Input: part model. Units: mm. Frame: model coordinates. Face numbers are marked on the shaded views. A direction names the side the tool comes from. Give positions to 0.01 mm unless a question says otherwise; leave off trailing zeros. Loops run counter-clockwise (first coordinate to the right, second up) from the corner with the lowest first, then second, coordinate; pieces in that order, holes last. Notation, with made-up numbers: (-10.75, -21.5) -> (30.25, -21.5) arc R18 ccw to (30.25, 5.5) -> close; hole circle Ø10 at (-32.5, -28). An arc over 180 degrees is marked (long way). Use CSV: the item, a comma, the result in double quotes.
```python
from build123d import *

# Parameters (mm, degrees)
BOSS_EXTRUDE1_DEPTH  = 2.54
SKETCH2_R            = 1.27
CUT_EXTRUDE1_DEPTH   = 5.334
SKETCH3_W            = 13.462
SKETCH3_H            = 27.94
BOSS_EXTRUDE2_DEPTH  = 2.54
BOSS_EXTRUDE3_DEPTH  = 13.462
BOSS_EXTRUDE7_DEPTH  = 1.27
BOSS_EXTRUDE12_DEPTH = 1.27


with BuildPart() as part:
    # Sketch1 → Boss-Extrude1 (new body)
    with BuildSketch(Plane(origin=(0, 0, 0), x_dir=(1, 0, 0), z_dir=(0, 1, 0))):
        Polygon((0, 0), (6.731, 0), (6.731, 38.1), (-6.731, 38.1), (-6.731, 0), align=None)
    extrude(amount=BOSS_EXTRUDE1_DEPTH)

    # Sketch2 → Cut-Extrude1 (cut)
    with BuildSketch(Plane(origin=(0, 2.54, 0), x_dir=(1, 0, 0), z_dir=(0, 1, 0))):
        with Locations(Location((0, 25.429147729, 0), (0, 0, 270))):
            Circle(SKETCH2_R)
        with Locations(Location((0, 12.776292729, 0), (0, 0, 270))):
            Circle(SKETCH2_R)
    extrude(amount=-CUT_EXTRUDE1_DEPTH, mode=Mode.SUBTRACT)

    # Sketch3 → Boss-Extrude2 (add)
    with BuildSketch(Plane.XY):
        with Locations((0, -11.43)):
            Rectangle(SKETCH3_W, SKETCH3_H)
    extrude(amount=-BOSS_EXTRUDE2_DEPTH)

    # Sketch4 → Boss-Extrude3 (add)
    with BuildSketch(Plane.ZY.offset(6.731)):
        with BuildLine():
            Line((0, -25.4), (-2.54, -25.4))
            ThreePointArc((-2.54, -25.4), (9.398, -37.338), (21.336, -25.4))
            Line((21.336, -25.4), (18.796, -25.4))
            ThreePointArc((18.796, -25.4), (9.398, -34.798), (0, -25.4))
        make_face()
    extrude(amount=-BOSS_EXTRUDE3_DEPTH)

    # Sketch8 → Boss-Extrude7 (add)
    with BuildSketch(Plane(origin=(6.731, 0, 0), x_dir=(0, 0, -1), z_dir=(1, 0, 0))):
        Polygon((2.54, -22.86), (20.32, 0), (12.400973841, 0), (2.54, -12.678394938), align=None)
    extrude(amount=-BOSS_EXTRUDE7_DEPTH)

    # Sketch9 → Boss-Extrude12 (add)
    with BuildSketch(Plane.ZY.offset(6.731)):
        Polygon((-2.54, -12.678394938), (-2.54, -22.86), (-20.32, 0), (-12.400973841, 0), align=None)
    extrude(amount=-BOSS_EXTRUDE12_DEPTH)


solid = part.part
```
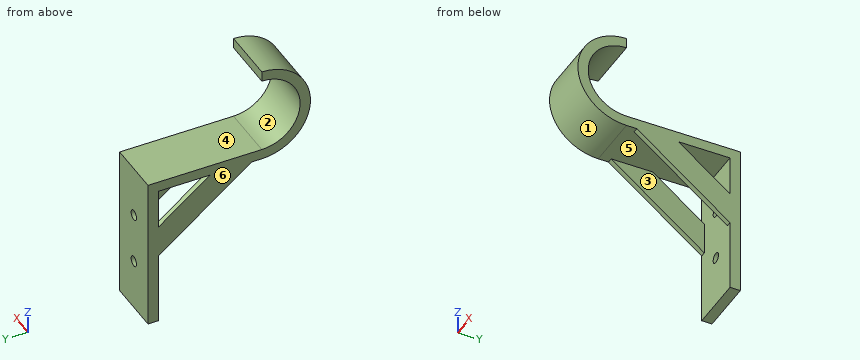
1) Reachability of the marked faces 5 and 6 from +Z, -Z, +X, -X, +Y, -Y: full face, straight path, thin tool, end or side. Return the list, or none.
From the geometry:
face 5,"none"
face 6,"+Z, -Z, -X, +Y, -Y"
2) Contact query for flat-ended pins moving along their axis: pin 1 (8 mm diameter, centred on x = -4, y = -16, fed in from -Z); pin 2 (1.5 mm diameter, centred on x = 0.5, z = 9, fed in from +Y); pin 3 (8 mm diameter, centred on x = 5, y = -9, fed in from -Z). Output: stop coordinate, or through.
From the geometry:
pin 1,"stops at z = -10.77"
pin 2,"stops at y = -34.73"
pin 3,"stops at z = -16.41"
3) Mould query, pull axis Z, two halves, no side actions, for the marked faces 1, 2, 3 and 4. Classes: pulls with the +Z half, pulls with the -Z half, needs draft (parallel to the pull), parting line crosses it, or undercut.
From the geometry:
face 1,"parting line crosses it"
face 2,"undercut"
face 3,"needs draft"
face 4,"pulls with the +Z half"
4) Section query D-D (y = -16.5). Return loops of the section in (x, z).
From the geometry:
outline,"(-6.73, -7.49) -> (-5.46, -7.49) -> (-5.46, -2.54) -> (5.46, -2.54) -> (5.46, -7.49) -> (6.73, -7.49) -> (6.73, 0) -> (-6.73, 0) -> close"
5) Section query B-B (y = -26.5). Return loops of the section in (x, z), then the cut area to 3 significant figures.
From the geometry:
outline,"(-6.73, -2.49) -> (6.73, -2.49) -> (6.73, 0.06) -> (-6.73, 0.06) -> close; (-6.73, 18.73) -> (6.73, 18.73) -> (6.73, 21.29) -> (-6.73, 21.29) -> close"
area,"68.8 mm^2"
6) Section query A-A (x = 0). Return loops of the section in (y, z).
From the geometry:
outline,"(-25.4, -2.54) -> (0, -2.54) -> (0, -11.51) -> (2.54, -11.51) -> (2.54, 0) -> (-25.4, 0) arc R9.4 cw to (-25.4, 18.8) -> (-25.4, 21.34) arc R11.94 ccw to start; (0, -38.1) -> (2.54, -38.1) -> (2.54, -26.7) -> (0, -26.7) -> close; (0, -24.16) -> (2.54, -24.16) -> (2.54, -14.05) -> (0, -14.05) -> close"
7) Section query C-C (z = -26). Return loops of the section in (x, y), then the cut area to 3 significant figures.
From the geometry:
outline,"(-6.73, 0) -> (-1.13, 0) -> (-1.13, 2.54) -> (-6.73, 2.54) -> close; (1.13, 0) -> (6.73, 0) -> (6.73, 2.54) -> (1.13, 2.54) -> close"
area,"28.4 mm^2"
8) Ray query, line 1 (Z direction, x = 4.75, y = -16); line 2 (Y direction, x = 2.5, z = -31); line 3 (Z direction, x = -2.75, y = -25.5). Return the intervals inside material, ascending.
From the geometry:
line 1,"z = -2.54 to 0"
line 2,"y = 0 to 2.54"
line 3,"z = -2.54 to 0, 18.8 to 21.34"
